Read the model definition and answer for the solid it produces. Units are mm, in the model's axes. A direction names the side the tool comes from. Give positions to 0.01 mm unless a question says otherwise; leave off trailing zeros. Loops run counter-clockwise (first coordinate to the right, second up) from the corner with the lowest first, then second, coordinate; pieces in that order, holes last. Notation, with made-up numbers: (23.25, 67) -> (31.25, 67) arc R19 cw to (31.25, 88) -> close; hole circle Ø11 at (30.25, 23.25). An arc over 180 degrees is marked (long way). Return JSON: item names as keys, results as strings. Group by question number.
from build123d import *

# Parameters (mm, degrees)
SKETCH1_W           = 64
SKETCH1_H           = 70
BOSS_EXTRUDE1_DEPTH = 2
SKETCH2_W           = 64
SKETCH2_H           = 70
BOSS_EXTRUDE2_DEPTH = 40
SKETCH3_R           = 2.25
SKETCH3_R_2         = 0.9
BOSS_EXTRUDE3_DEPTH = 5
SKETCH4_W           = 52
SKETCH4_H           = 40
CUT_EXTRUDE1_DEPTH  = 2
SKETCH5_R           = 1
CUT_EXTRUDE4_DEPTH  = 4
CUT_EXTRUDE5_DEPTH  = 2.3
SKETCH7_R           = 1.4
CUT_EXTRUDE6_DEPTH  = 12
CUT_EXTRUDE7_REACH  = 105.73
SKETCH8_W           = 12
SKETCH8_H           = 27


with BuildPart() as part:
    # Sketch1 → Boss-Extrude1 (new body)
    with BuildSketch(Plane(origin=(0, 0, 0), x_dir=(1, 0, 0), z_dir=(0, 1, 0))):
        with Locations((32, -35)):
            Rectangle(SKETCH1_W, SKETCH1_H)
    extrude(amount=BOSS_EXTRUDE1_DEPTH)

    # Sketch2 → Boss-Extrude2 (add)
    with BuildSketch(Plane(origin=(0, 2, 0), x_dir=(1, 0, 0), z_dir=(0, 1, 0))):
        with Locations((32, -35)):
            Rectangle(SKETCH2_W, SKETCH2_H)
        Polygon((14, -2), (57, -2), (57, -9), (62, -9), (62, -61), (57, -61), (57, -68), (14, -68), (14, -62.5), (2, -62.5), (2, -7.5), (14, -7.5), align=None, mode=Mode.SUBTRACT)
    extrude(amount=BOSS_EXTRUDE2_DEPTH)

    # Sketch3 → Boss-Extrude3 (add)
    # profile 1 of 4: a face of its own
    with BuildSketch(Plane(origin=(0, 2, 0), x_dir=(1, 0, 0), z_dir=(0, 1, 0))):
        with Locations(Location((21, -58.75, 0), (0, 0, 270))):
            Circle(SKETCH3_R)
        with Locations(Location((21, -58.75, 0), (0, 0, 270))):
            Circle(SKETCH3_R_2, mode=Mode.SUBTRACT)
    # profile 2 of 4: a face of its own
    with BuildSketch(Plane(origin=(0, 2, 0), x_dir=(1, 0, 0), z_dir=(0, 1, 0))):
        with Locations(Location((46, -58.75, 0), (0, 0, 270))):
            Circle(SKETCH3_R)
        with Locations(Location((46, -58.75, 0), (0, 0, 270))):
            Circle(SKETCH3_R_2, mode=Mode.SUBTRACT)
    # profile 3 of 4: a face of its own
    with BuildSketch(Plane(origin=(0, 2, 0), x_dir=(1, 0, 0), z_dir=(0, 1, 0))):
        with Locations(Location((21, -11.25, 0), (0, 0, 270))):
            Circle(SKETCH3_R)
        with Locations(Location((21, -11.25, 0), (0, 0, 270))):
            Circle(SKETCH3_R_2, mode=Mode.SUBTRACT)
    # profile 4 of 4: a face of its own
    with BuildSketch(Plane(origin=(0, 2, 0), x_dir=(1, 0, 0), z_dir=(0, 1, 0))):
        with Locations(Location((46, -11.25, 0), (0, 0, 270))):
            Circle(SKETCH3_R)
        with Locations(Location((46, -11.25, 0), (0, 0, 270))):
            Circle(SKETCH3_R_2, mode=Mode.SUBTRACT)
    extrude(amount=BOSS_EXTRUDE3_DEPTH)

    # Sketch4 → Cut-Extrude1 (cut)
    with BuildSketch(Plane(origin=(64, 0, 0), x_dir=(0, 0, -1), z_dir=(1, 0, 0))):
        with Locations((-35, 22)):
            Rectangle(SKETCH4_W, SKETCH4_H)
    extrude(amount=-CUT_EXTRUDE1_DEPTH, mode=Mode.SUBTRACT)

    # Sketch5 → Cut-Extrude4 (cut)
    with BuildSketch(Plane.ZY.offset(-57)):
        with Locations((7, 40)):
            Circle(SKETCH5_R)
        with Locations((7, 4)):
            Circle(SKETCH5_R)
        with Locations((63, 4)):
            Circle(SKETCH5_R)
        with Locations((63, 40)):
            Circle(SKETCH5_R)
    extrude(amount=-CUT_EXTRUDE4_DEPTH, mode=Mode.SUBTRACT)

    # Sketch6 → Cut-Extrude5 (cut)
    with BuildSketch(Plane(origin=(0, 42, 0), x_dir=(1, 0, 0), z_dir=(0, 1, 0))):
        Polygon((3.212435565, -2), (2.606217783, -0.95), (1.393782217, -0.95), (0.787564435, -2), (1.393782217, -3.05), (2.606217783, -3.05), align=None)
        Polygon((3.212435565, -68), (2.606217783, -66.95), (1.393782217, -66.95), (0.787564435, -68), (1.393782217, -69.05), (2.606217783, -69.05), align=None)
        Polygon((60.787564435, -68), (61.393782217, -69.05), (62.606217783, -69.05), (63.212435565, -68), (62.606217783, -66.95), (61.393782217, -66.95), align=None)
        Polygon((60.787564435, -2), (61.393782217, -3.05), (62.606217783, -3.05), (63.212435565, -2), (62.606217783, -0.95), (61.393782217, -0.95), align=None)
    extrude(amount=-CUT_EXTRUDE5_DEPTH, mode=Mode.SUBTRACT)

    # Sketch7 → Cut-Extrude6 (cut)
    with BuildSketch(Plane(origin=(14, 0, 0), x_dir=(0, 0, -1), z_dir=(1, 0, 0))):
        with Locations((-65.5, 37.5)):
            Circle(SKETCH7_R)
        with Locations((-4.5, 37.5)):
            Circle(SKETCH7_R)
        with Locations((-65.5, 6.5)):
            Circle(SKETCH7_R)
        with Locations((-4.5, 6.5)):
            Circle(SKETCH7_R)
    extrude(amount=-CUT_EXTRUDE6_DEPTH, mode=Mode.SUBTRACT)

    # Cut-Extrude7: up to this face of the body (flat: up to its plane)
    cut_extrude7_end = Plane(part.part.faces().sort_by_distance((35.5, 22, 2))[0])
    # Sketch8 → Cut-Extrude7 (cut, up to the picked face)
    with BuildSketch(Plane.XY.offset(70), mode=Mode.PRIVATE) as cut_extrude7_sk1:
        with Locations((8, 22)):
            Rectangle(SKETCH8_W, SKETCH8_H)
    cut_extrude7_tool1 = split(extrude(cut_extrude7_sk1.sketch, amount=-CUT_EXTRUDE7_REACH, mode=Mode.PRIVATE), bisect_by=cut_extrude7_end, keep=Keep.BOTH, mode=Mode.PRIVATE)
    add(cut_extrude7_tool1.solids().sort_by(Axis((8, 22, 70), (0, 0, -1)))[0], mode=Mode.SUBTRACT)


solid = part.part
1. Section A-A on x = 5.5 is taken. Determine the outline of the cut face in (y, z).
2. Which of the six approach directions +Z, -Z, +X, -X, +Y, -Y give full straight-line access (tool end or side, diameter ignored) to faces 4 (the flat face through (2, 39.7, 68)), 5 (the flat face through (14, 22, 69)), 6 (the flat face through (61, 22, 9)), 7 (the flat face through (2, 22, 36))?
3. Section C-C on y = 32 is taken. Determine the outline of the cut face in (x, z).
4. Section D-D on z = 65.5 is taken. Determine the outline of the cut face in (x, y), then the cut area to 3 significant figures.
5. Straight lines are drawn through the part: line 1 (Z direction, x = 53, y = 39.5); line 2 (X direction, y = 25, z = 5); line 3 (Z direction, x = 60.5, y = 3.5). For each, find the intervals that lie inside material, in ascending order. Write a range as from..to.
6. Determine the mould class of faces 1 (the flat face through (21, 7, 60)), 2 (the flat face through (64, 1, 38)), 3 (the cylindrical face through (8.084, 6.921, 64.165)) for opening direction X: pulls with the +X half, pulls with the -X half, needs draft (parallel to the pull), parting line crosses it, or undercut.
7. Section B-B on y = 4 is taken. State how many separate pieces and enclosed holes the cut face has, then the cut area to 3 significant figures.
8. Flat-ended cylindrical pins translate along their axes: pin 1 Ø1.4 at (x, z) = (46, 58.75) entering from +Y; pin 2 Ø4 at (x, y) = (31.5, 7) entering from -Z; pin 3 Ø2 at (x, z) = (21, 12.5) entering from +Y; pin 4 Ø1 at (x, y) = (10, 19.5) entering from +Z. Find the tip coordinate at first contact, or state that the pin passes through.
Completed:
{
 "1": {"outline": "(0, 0) -> (42, 0) -> (42, 7.5) -> (35.5, 7.5) -> (35.5, 2) -> (8.5, 2) -> (8.5, 7.5) -> (2, 7.5) -> (2, 62.5) -> (8.5, 62.5) -> (8.5, 70) -> (0, 70) -> close; (35.5, 62.5) -> (42, 62.5) -> (42, 70) -> (35.5, 70) -> close; hole circle Ø2.8 at (6.5, 4.5); hole circle Ø2.8 at (6.5, 65.5); hole circle Ø2.8 at (37.5, 4.5); hole circle Ø2.8 at (37.5, 65.5)"},
 "2": {"face 4": "+Y", "face 5": "+Z", "face 6": "+X, +Y", "face 7": "none"},
 "3": {"outline": "(0, 0) -> (64, 0) -> (64, 9) -> (57, 9) -> (57, 2) -> (2, 2) -> (2, 70) -> (0, 70) -> close; (14, 68) -> (57, 68) -> (57, 61) -> (64, 61) -> (64, 70) -> (14, 70) -> close"},
 "4": {"outline": "(0, 0) -> (64, 0) -> (64, 42) -> (57, 42) -> (57, 2) -> (14, 2) -> (14, 5.1) -> (2, 5.1) -> (2, 7.9) -> (14, 7.9) -> (14, 8.5) -> (2, 8.5) -> (2, 35.5) -> (14, 35.5) -> (14, 36.1) -> (2, 36.1) -> (2, 38.9) -> (14, 38.9) -> (14, 42) -> (0, 42) -> close", "area": "577 mm²"},
 "5": {"line 1": "z = 0..2, 68..70", "line 2": "x = 0..2, 57..64", "line 3": "z = 0..6.13, 7.87..9, 61..62.13, 63.87..70"},
 "6": {"face 1": "needs draft", "face 2": "pulls with the +X half", "face 3": "undercut"},
 "7": {"separate pieces": "5", "enclosed holes": "4", "area": "655 mm²"},
 "8": {"pin 1": "stops at y = 2", "pin 2": "stops at z = 0", "pin 3": "stops at y = 7", "pin 4": "stops at z = 2"}
}
